```python
from build123d import *

# Parameters (mm, degrees)
EXTRUDE_2_DEPTH = 3


with BuildPart() as part:
    # 草图1 → 凸台-拉伸2 (new body)
    with BuildSketch(Plane.XY):
        with BuildLine():
            Line((-8.443741515, -3.928837448), (8.443741515, -3.928837448))
            ThreePointArc((8.443741515, -3.928837448), (9.857955078, -3.34305101), (10.443741515, -1.928837448))
            Line((10.443741515, -1.928837448), (10.443741515, 1.702434927))
            Line((10.443741515, 1.702434927), (10.443741515, 18.702434927))
            ThreePointArc((10.443741515, 18.702434927), (11.322421172, 20.823755271), (13.443741515, 21.702434927))
            Line((13.443741515, 21.702434927), (42, 21.702434927))
            ThreePointArc((42, 21.702434927), (44.121320344, 22.581114584), (45, 24.702434927))
            Line((45, 24.702434927), (45, 43.196509927))
            ThreePointArc((45, 43.196509927), (44.121320344, 45.31783027), (42, 46.196509927))
            Line((42, 46.196509927), (-42, 46.196509927))
            ThreePointArc((-42, 46.196509927), (-44.121320344, 45.31783027), (-45, 43.196509927))
            Line((-45, 43.196509927), (-45, 24.702434927))
            ThreePointArc((-45, 24.702434927), (-44.121320344, 22.581114584), (-42, 21.702434927))
            Line((-42, 21.702434927), (-13.443741515, 21.702434927))
            ThreePointArc((-13.443741515, 21.702434927), (-11.322421172, 20.823755271), (-10.443741515, 18.702434927))
            Line((-10.443741515, 18.702434927), (-10.443741515, 1.702434927))
            Line((-10.443741515, 1.702434927), (-10.443741515, -1.928837448))
            ThreePointArc((-10.443741515, -1.928837448), (-9.857955078, -3.34305101), (-8.443741515, -3.928837448))
        make_face()
        with BuildLine():
            Line((-7.430734656, 1.6), (7.569265344, 1.6))
            ThreePointArc((7.569265344, 1.6), (9.169265344, 0), (7.569265344, -1.6))
            Line((7.569265344, -1.6), (-7.430734656, -1.6))
            ThreePointArc((-7.430734656, -1.6), (-9.030734656, 0), (-7.430734656, 1.6))
        make_face(mode=Mode.SUBTRACT)
        with BuildLine():
            Line((36.883924739, 25.196509927), (-36.883924739, 25.196509927))
            ThreePointArc((-36.883924739, 25.196509927), (-38.209103575, 26.501622059), (-37.4430933, 28.196509927))
            Line((-37.4430933, 28.196509927), (37.4430933, 28.196509927))
            ThreePointArc((37.4430933, 28.196509927), (38.209103575, 26.501622059), (36.883924739, 25.196509927))
        make_face(mode=Mode.SUBTRACT)
    extrude(amount=EXTRUDE_2_DEPTH)


solid = part.part
```
Design review of the part built by this model. Coordinates are the model's own, in mm. A direction names the side the tool comes from. Coordinates: 2 decimals unless noted, no trailing zeros. Order: outer loops, then holes, each group sorted by start corner. A loop starts at its lowest first (then second) coordinate and runs counter-clockwise, first axis right, second up. Notation, with made-up numbers: M 21,66 L 61,66 A31 cw 61,104 Z; hole C 21.25,87.25 d9. An arc over 180 degrees is marked long. Answer as a JSON object with one key per item and string values. Group by question number.
1) For pin 1 (0.9 mm diameter, centred on x = -27.5, z = 1.5, fed in from -Y), flat-tipped, find the tip position at first contact; note if it passes through.
2) Add section A-A, the plane x = -36. Write out the cut boundary in (y, z).
3) Mouldability with a two-part tool opening along X and no side actions: class faces 5 (the flat face through (-10.444, 9, 1)), 6 (the cylindrical face through (9.17, 0.04, 1.48)), 7 (the flat face through (-1, 33, 0)) as pulls with the +X half, pulls with the -X half, needs draft (parallel to the pull), parting line crosses it, or undercut.
4) Add section C-C, the plane y = 0. Write out the cut boundary in (x, z), then the cut area to 3 significant figures.
5) Add section D-D, the plane x = 1.5. Write out the cut boundary in (y, z).
6) Wall thickness on L1, parallel to Y at x = -1, z = 1.65; L2, parallel to Y at x = -33.5, z = 1.7; L3, parallel to X at y = 13, z = 1.15: over which ranges is each line inside the solid? List them lowest first.
7) Add section B-B, the plane z = 0.9. Write out the cut boundary in (x, y).
8) Tool access review of faces 1 (the flat face through (-28, 21.702, 1)), 2 (the cylindrical face through (44.145, 45.294, 1.479)), 3 (the flat face through (10.444, 8, 1)), 4 (the cylindrical face through (-9.03, -0.04, 1.48)): name each direction out of +Z, -Z, +X, -X, +Y, -Y from which nothing blocks a thin tool from reaching the whole face with its end or side.
Computed values:
{
 "1": {"pin 1": "stops at y = 21.7"},
 "2": {"outline": "M 21.7,0 L 25.2,0 L 25.2,3 L 21.7,3 Z; M 28.2,0 L 46.2,0 L 46.2,3 L 28.2,3 Z"},
 "3": {"face 5": "pulls with the -X half", "face 6": "undercut", "face 7": "needs draft"},
 "4": {"outline": "M -10.44,0 L -9.03,0 L -9.03,3 L -10.44,3 Z; M 9.17,0 L 10.44,0 L 10.44,3 L 9.17,3 Z", "area": "8.06 mm^2"},
 "5": {"outline": "M -3.93,0 L -1.6,0 L -1.6,3 L -3.93,3 Z; M 1.6,0 L 25.2,0 L 25.2,3 L 1.6,3 Z; M 28.2,0 L 46.2,0 L 46.2,3 L 28.2,3 Z"},
 "6": {"L1": "y = -3.93 to -1.6, 1.6 to 25.2, 28.2 to 46.2", "L2": "y = 21.7 to 25.2, 28.2 to 46.2", "L3": "x = -10.44 to 10.44"},
 "7": {"outline": "M -45,24.7 A3 ccw -42,21.7 L -13.44,21.7 A3 cw -10.44,18.7 L -10.44,-1.93 A2 ccw -8.44,-3.93 L 8.44,-3.93 A2 ccw 10.44,-1.93 L 10.44,18.7 A3 cw 13.44,21.7 L 42,21.7 A3 ccw 45,24.7 L 45,43.2 A3 ccw 42,46.2 L -42,46.2 A3 ccw -45,43.2 Z; hole M -37.44,28.2 A1.63 ccw -36.88,25.2 L 36.88,25.2 A1.63 ccw 37.44,28.2 Z; hole M -7.43,-1.6 L 7.57,-1.6 A1.6 ccw 7.57,1.6 L -7.43,1.6 A1.6 ccw Z"},
 "8": {"face 1": "+Z, -Z, -X, -Y", "face 2": "+Z, -Z, +X, +Y", "face 3": "+Z, -Z, +X, -Y", "face 4": "+Z, -Z"}
}
